```python
from build123d import *

# Parameters (mm, degrees)
PLATE_THICKNESS_3MM_DEPTH = 3
SKETCH_1_W                = 3.5
SKETCH_1_H                = 3
EXTRUDE_2_DEPTH           = 3


with BuildPart() as part:
    # Sketch1 → Plate_thickness_3mm (new body)
    with BuildSketch(Plane.XY):
        Polygon((21.57, 0), (0, 0), (0, 20), (3, 20), (3, 40), (0, 40), (0, 60), (10.785, 60), (10.785, 63), (13.785, 63), (13.785, 60), (21.57, 60), (21.57, 40), (24.57, 40), (24.57, 20), (21.57, 20), align=None)
    extrude(amount=PLATE_THICKNESS_3MM_DEPTH)

    # 草图1 → 凸台-拉伸2 (add)
    with BuildSketch(Plane.XY.offset(3)):
        with Locations((9.035, 61.5)):
            Rectangle(SKETCH_1_W, SKETCH_1_H)
        with Locations((15.535, 61.5)):
            Rectangle(SKETCH_1_W, SKETCH_1_H)
    extrude(amount=-EXTRUDE_2_DEPTH)


solid = part.part
```
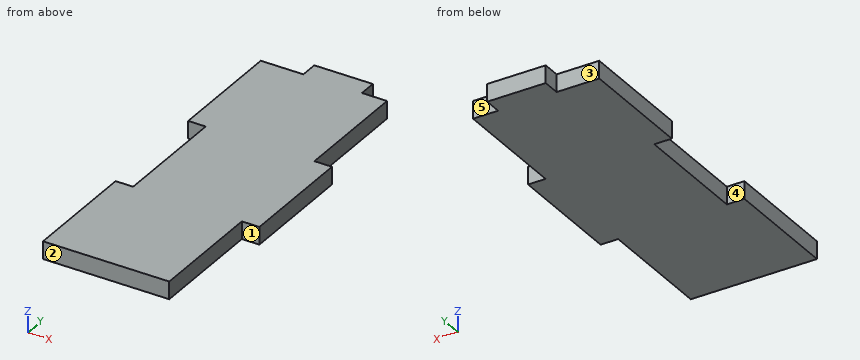
Work out the finished part from the listing and answer in its coordinate system (mm). Face numbers are marked on the shaded views. A direction names the side the tool comes from. Round coordinates to 2 decimals unless told otherwise and drop trailing zeros. Loops run counter-clockwise (first coordinate to the right, second up) from the corner with the lowest first, then second, coordinate; pieces in that order, holes last.
(1) Find the intervals of material crossed by L1, parallel to Y at x = 20.5, z = 2.2; L2, parallel to X at y = 3.5, z = 0.65; L3, parallel to X at y = 39, z = 0.4, in increasing order.
Computed values:
L1: y = 0 to 60
L2: x = 0 to 21.57
L3: x = 3 to 24.57
(2) The part is cut by section B-B, the plane y = 9.5. Give the vertices of the cut face in (x, z).
Computed values:
outline: (0, 0) - (21.57, 0) - (21.57, 3) - (0, 3) - close
(3) The part is cut by section A-A, the plane z = 0.5. Give the vertices of the cut face in (x, y) (3 decimals).
Computed values:
outline: (0, 0) - (21.57, 0) - (21.57, 20) - (24.57, 20) - (24.57, 40) - (21.57, 40) - (21.57, 60) - (17.285, 60) - (17.285, 63) - (7.285, 63) - (7.285, 60) - (0, 60) - (0, 40) - (3, 40) - (3, 20) - (0, 20) - close
(4) The part is cut by section C-C, the plane x = 22.25. Give the vertices of the cut face in (y, z).
Computed values:
outline: (20, 0) - (40, 0) - (40, 3) - (20, 3) - close
(5) For the marked faces 1, 2, 3, 4 and 5, determine the directions among +Z, -Z, +X, -X, +Y, -Y from which every point of the face is accessible in a straight line to the end or side of a thin tool.
Computed values:
face 1: +Z, -Z, +X, -Y
face 2: +Z, -Z, +X, -X, -Y
face 3: +Z, -Z, -X, +Y
face 4: +Z, -Z, -X
face 5: +Z, -Z, +X, +Y
(6) Each of these flat-tipped pins is pushed along its axis until it touches: P1, Ø1.5, axis at x = 3.5, z = 1, coming from the +Y side; P2, Ø0.9, axis at y = 29, z = 2, coming from the -X side; P3, Ø0.9, axis at y = 61.5, z = 2, coming from the -X side (3 decimals). Where does it stop, or does it pass through?
Computed values:
P1: stops at y = 60
P2: stops at x = 3
P3: stops at x = 7.285
